Input: part model. Units: mm. Frame: model coordinates. A direction names the side the tool comes from. Round coordinates to 2 decimals unless told otherwise and drop trailing zeros. Write each loop counter-clockwise with the first axis right and the second up, starting at its lowest first coordinate (ties: lowest second). Pieces come first, ordered by that corner, then holes. Notation, with made-up numbers: (37.25, -26.5) -> (46.25, -26.5) arc R18 cw to (46.25, 2.5) -> close; hole circle Ø6 at (-32, 1.5). An arc over 180 degrees is marked (long way). Use CSV: the item, a comma, the result in double quotes.
```python
from build123d import *

# Parameters (mm, degrees)
F0_W     = 5
F0_H     = 15
F2_R     = 3
F2_R_2   = 1.25
F3_DEPTH = 5
F5_DEPTH = 5
F6_W     = 12.5
F6_H     = 10
F7_DEPTH = 9
F8_W     = 12.5
F8_H     = 9.5
F9_DEPTH = 3


with BuildPart() as f1:
    # F0 (on Front) → F1 (revolve)
    with BuildSketch(Plane.XZ):
        with Locations((2.5, 7.5)):
            Rectangle(F0_W, F0_H)
    revolve(axis=Axis((0, 0, 7.5), (0, 0, 1)))

    # F2 (on face) → F3 (cut)
    with BuildSketch(Plane(origin=(0, 0, 0), x_dir=(1, 0, 0), z_dir=(0, 0, -1))):
        Circle(F2_R)
        Circle(F2_R_2, mode=Mode.SUBTRACT)
    extrude(amount=-F3_DEPTH, mode=Mode.SUBTRACT)

    # F4 (on Front) → F5 (join, symmetric)
    with BuildSketch(Plane.XZ):
        Polygon((-6.25, 24), (-5, 15), (5, 15), (6.25, 24), align=None)
    extrude(amount=F5_DEPTH, both=True)

    # F6 (on face) → F7 (join)
    with BuildSketch(Plane.XY.offset(24)):
        Rectangle(F6_W, F6_H)
    extrude(amount=F7_DEPTH)

    # F8 (on face) → F9 (join)
    with BuildSketch(Plane.XY.offset(33)):
        with Locations((0, -0.75)):
            Rectangle(F8_W, F8_H)
    extrude(amount=F9_DEPTH)


solid = f1.part
```
Item 1: Section query D-D on z = 20. Return the cut outline in (x, y), plus the area to 3 significant figures.
Worked answers:
outline,"(-5.69, -5) -> (5.69, -5) -> (5.69, 5) -> (-5.69, 5) -> close"
area,"114 mm²"
Item 2: Pull-direction query (Y, two-part tool) for faces 1 (the face through (-0.27, 1.22, 2.46)), 2 (the face through (-3, 0, 2)), 3 (the face through (0, 5, 24)), 4 (the face through (0, -5.5, 34)); classes: +Y half, -Y half, draft (parallel to the pull), parting line (faces both ways), or undercut.
Worked answers:
face 1,"undercut"
face 2,"undercut"
face 3,"+Y half"
face 4,"-Y half"
Item 3: Section query B-B on y = -2. Return the cut outline in (x, z), plus the area to 3 significant figures.
Worked answers:
outline,"(-6.25, 24) -> (-5, 15) -> (-4.58, 15) -> (-4.58, 0) -> (-2.24, 0) -> (-2.24, 5) -> (2.24, 5) -> (2.24, 0) -> (4.58, 0) -> (4.58, 15) -> (5, 15) -> (6.25, 24) -> (6.25, 36) -> (-6.25, 36) -> close"
area,"366 mm²"
Item 4: Set-up query: faces 5 (the face through (-4, -4, 15)), 6 (the face through (-1.08, -4.88, 7.6)), 7 (the face through (0, -5, 24)), 8 (the face through (4, -4, 15)). Return all of +Z, -Z, +X, -X, +Y, -Y with unobstructed straight access to the full face (end or side cutting, diameter ignored); none if empty.
Worked answers:
face 5,"-Z, -X, -Y"
face 6,"-Z"
face 7,"-Z, +X, -X, -Y"
face 8,"-Z, +X, -Y"
Item 5: First-contact query: pin 1 Ø0.8 at (x, y) = (-1.5, 4.5) entering from +Z; pin 2 Ø0.9 at (x, z) = (2.5, 34) entering from +Y; pin 3 Ø3 at (y, z) = (0, 18) entering from -X (3 decimals). Flat tips, straight axial feed; report the tip coordinate or a pass-through.
Worked answers:
pin 1,"stops at z = 33"
pin 2,"stops at y = 4"
pin 3,"stops at x = -5.625"
Item 6: Section query A-A on z = 4. Return the cut outline in (x, y), plus the area to 3 significant figures.
Worked answers:
outline,"circle Ø10 at (0, 0); circle Ø2.5 at (0, 0); hole circle Ø6 at (0, 0)"
area,"55.2 mm²"
Item 7: Section query C-C on x = -3.5. Return the cut outline in (y, z).
Worked answers:
outline,"(-5.5, 33) -> (-5, 33) -> (-5, 15) -> (-3.57, 15) -> (-3.57, 0) -> (3.57, 0) -> (3.57, 15) -> (5, 15) -> (5, 33) -> (4, 33) -> (4, 36) -> (-5.5, 36) -> close"
Item 8: Line query: line 1 (Y direction, x = 0, z = 1.75); line 2 (X direction, y = -0.25, z = 4); line 3 (Y direction, x = 2.25, z = 21). Output: solid intervals per line, ascending.
Worked answers:
line 1,"y = -5 to -3, -1.25 to 1.25, 3 to 5"
line 2,"x = -4.99 to -2.99, -1.22 to 1.22, 2.99 to 4.99"
line 3,"y = -5 to 5"
